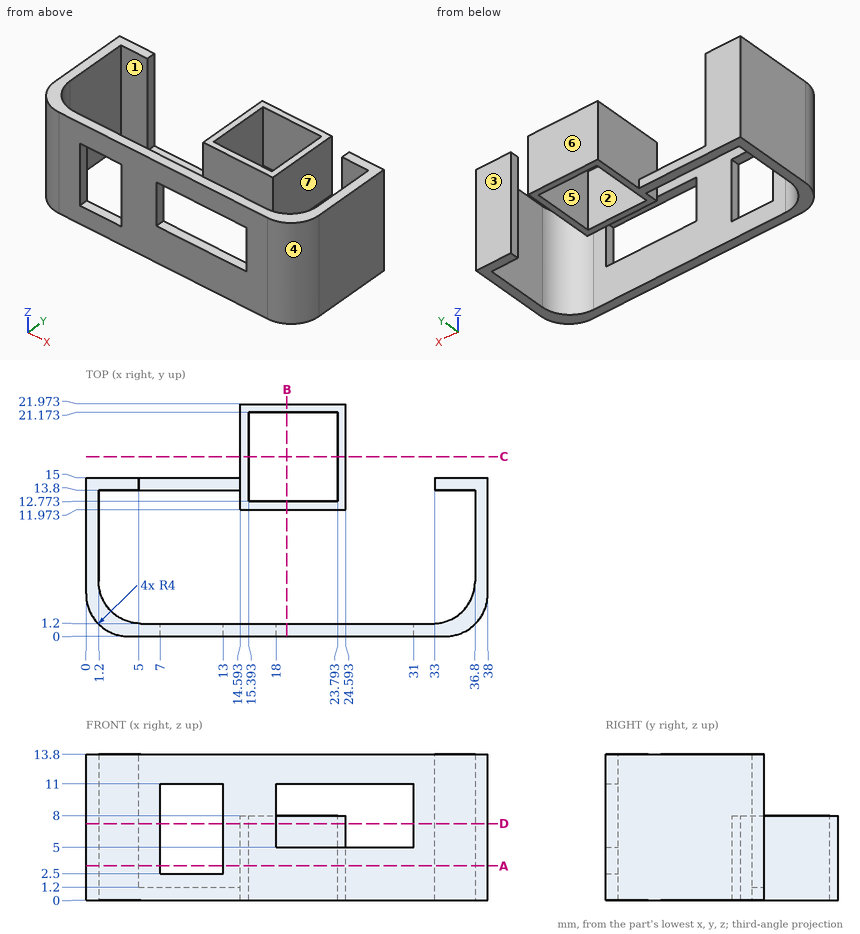
Could you check a few things on this drawing? It's one solid part, dimensions in mm from its lowest x, y, z. A direction names the side the tool comes from. Round coordinates to 2 decimals unless told otherwise and drop trailing zeros. Write each loop counter-clockwise with the first axis right and the second up, starting at its lowest first coordinate (ties: lowest second). Pieces come first, ordered by that corner, then holes. Notation, with made-up numbers: (-4, -26) -> (44, -26) arc R18 cw to (44, -5) -> close; hole circle Ø3 at (1, 71.25). An arc over 180 degrees is marked (long way). Use one line per item in the form item = value. Start each with the question number.
Q1. We'd pull the mould along X, two halves only. Please class the marked faces 1, 2, 3 and 4: +X half, -X half, draft (parallel to the pull), parting line (faces both ways), or undercut.
Q2. Imagine slicing it at D-D (z = 7.25). Count the separate pieces of the cut face and the enclosed holes in it.
Q3. Imagine slicing it at A-A (z = 3.25). Please give me the cut outline in (x, y).
Q4. Which directions (+Z, -Z, +X, -X, +Y, -Y) give clear straight access to the entire face, cutting with the end or side of a thin tool? Please do the marked faces 5, 6 and 7.
Q5. I'm going to push flat-ended pins straight in: P1, Ø1.3, axis at y = 0.5, z = 7.5, coming from the +X side; P2, Ø5, axis at x = 17.5, y = 15, coming from the +Z side; P3, Ø1, axis at y = 2.5, z = 10.5, coming from the -X side. Where does each tip first touch, or does it pass through?
Q6. If I drill on probe 1 along X at (y, z) = (13.25, 5.75); probe 2 along Y at (x, z) = (16, 5.75); probe 3 along X at (y, z) = (6, 7.75), over which ranges is the centre line in solid material (lowest first)? Write a range as [from, to].
Q7. Imagine slicing it at B-B (x = 19). Please give me the cut outline in (y, z).
Q8. Imagine slicing it at C-C (y = 17). Please give me the cut outline in (x, z), then the cut area to 3 significant figures.
Worked out:
q1.face_1 = undercut
q1.face_2 = undercut
q1.face_3 = draft
q1.face_4 = +X half
q2.separate_pieces = 4
q2.enclosed_holes = 1
q3.outline = (0, 4) arc R4 ccw to (4, 0) -> (7, 0) -> (7, 1.2) -> (5.2, 1.2) arc R4 cw to (1.2, 5.2) -> (1.2, 13.8) -> (5, 13.8) -> (5, 15) -> (0, 15) -> close; (13, 0) -> (34, 0) arc R4 ccw to (38, 4) -> (38, 15) -> (33, 15) -> (33, 13.8) -> (36.8, 13.8) -> (36.8, 5.2) arc R4 cw to (32.8, 1.2) -> (13, 1.2) -> close; (14.59, 11.97) -> (24.59, 11.97) -> (24.59, 21.97) -> (14.59, 21.97) -> close; hole (15.39, 12.77) -> (23.79, 12.77) -> (23.79, 21.17) -> (15.39, 21.17) -> close
q4.face_5 = +Z, -Z
q4.face_6 = +Z, -Z, +X, -X, +Y
q4.face_7 = +Z, -Z, +Y
q5.P1 = 36.81
q5.P2 = 8
q5.P3 = 0.13
q6.probe_1 = [0, 1.2], [14.59, 15.39], [23.79, 24.59], [36.8, 38]
q6.probe_2 = [0, 1.2], [11.97, 12.77], [21.17, 21.97]
q6.probe_3 = [0, 1.2], [36.8, 38]
q7.outline = (0, 0) -> (1.2, 0) -> (1.2, 5) -> (0, 5) -> close; (0, 11) -> (1.2, 11) -> (1.2, 13.8) -> (0, 13.8) -> close; (11.97, 0) -> (12.77, 0) -> (12.77, 8) -> (11.97, 8) -> close; (21.17, 0) -> (21.97, 0) -> (21.97, 8) -> (21.17, 8) -> close
q8.outline = (14.59, 0) -> (15.39, 0) -> (15.39, 8) -> (14.59, 8) -> close; (23.79, 0) -> (24.59, 0) -> (24.59, 8) -> (23.79, 8) -> close
q8.area = 12.8 mm^2
